Could you check a few things on this model? Use its own coordinates, in mm. Face numbers are marked on the shaded views. Coordinates: 2 decimals unless noted, no trailing zeros. Loops run counter-clockwise (first coordinate to the right, second up) from the corner with the lowest first, then second, coordinate; pieces in that order, holes last.
1) Thinking about a two-plate mould opening in Y: for the marked faces 1, 2, 3 and 4, which applies, released by +Y, released by -Y, zero draft, split by the parting line, or undercut?
2) Imagine slicing it at C-C on x = 53. Please give me the cut outline in (y, z).
3) Imagine slicing it at B-B on z = 4.25. Give the number of separate pieces and of enclosed holes in the cut face, plus the area to 3 significant figures.
4) Will these pins go through, and if not, where does the flat tip stop? P1, Ø3, axis at x = -17.5, y = 19.5, coming from the +Z side; P2, Ø17, axis at x = 53, y = 0, coming from the +Z side.
5) Imagine slicing it at D-D on y = 9. Please give me the cut outline in (x, z), plus the area to 3 significant figures.
6) Imagine slicing it at A-A on y = 0. Please give me the cut outline in (x, z).
7) If I drill on line 1 along X through (y, z) = (-9.5, 6); line 2 along X through (y, z) = (6, 11); line 3 along Y through (x, z) = (1, 7.25), over which ranges is the centre line in solid material (lowest first)?
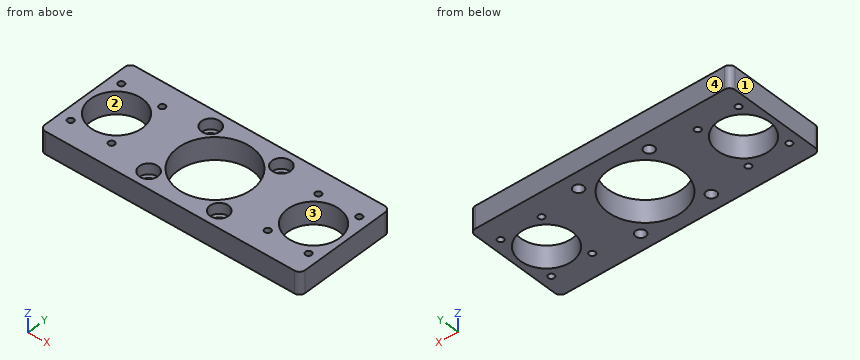
```python
from build123d import *

# Parameters (mm, degrees)
SKETCH_1_W                = 140
SKETCH_1_H                = 55
EXTRUDE_1_DEPTH           = 12
SKETCH_2_R                = 20
SKETCH_2_R_2              = 14
CUT_EXTRUDE_1_DEPTH       = 77.159372371
FILLET_1_R                = 3
HOLE_WIZARD_M4_1_D        = 3.3
HOLE_WIZARD_1_D           = 5.5
HOLE_WIZARD_1_CBORE_D     = 10
HOLE_WIZARD_1_CBORE_DEPTH = 5.7


with BuildPart() as part:
    # 草图1 → 凸台-拉伸1 (new body)
    with BuildSketch(Plane.XY):
        Rectangle(SKETCH_1_W, SKETCH_1_H)
    extrude(amount=EXTRUDE_1_DEPTH)

    # 草图2 → 切除-拉伸1 (cut, through all)
    with BuildSketch(Plane.XY.offset(12)):
        Circle(SKETCH_2_R)
        with Locations((-53, 0)):
            Circle(SKETCH_2_R_2)
        with Locations((53, 0)):
            Circle(SKETCH_2_R_2)
    extrude(amount=-CUT_EXTRUDE_1_DEPTH, mode=Mode.SUBTRACT)

    # 圆角1
    fillet_1_edges = [part.edges().sort_by_distance(p)[0] for p in [
        (70, -27.5, 6),
        (-70, -27.5, 6),
        (-70, 27.5, 6),
        (70, 27.5, 6),
    ]]
    fillet(fillet_1_edges, radius=FILLET_1_R)

    # M4 螺纹孔1 (through all)
    with Locations(Plane.XY.offset(12)):
        with Locations((-64, 15.5), (-42, 15.5), (-42, -15.5), (-64, -15.5), (42, -15.5), (64, -15.5), (64, 15.5), (42, 15.5)):
            Hole(HOLE_WIZARD_M4_1_D / 2)

    # 打孔尺寸(%根据)内六角圆柱头螺钉的类型1 (through all)
    with Locations(Plane.XY.offset(12)):
        with Locations((-19, 19), (19, 19), (19, -19), (-19, -19)):
            CounterBoreHole(HOLE_WIZARD_1_D / 2, HOLE_WIZARD_1_CBORE_D / 2, HOLE_WIZARD_1_CBORE_DEPTH)


solid = part.part
```
Filled in:
1. face 1: zero draft
1. face 2: undercut
1. face 3: undercut
1. face 4: released by +Y
2. outline: (-27.5, 0) - (-14, 0) - (-14, 12) - (-27.5, 12) - close; (14, 0) - (27.5, 0) - (27.5, 12) - (14, 12) - close
3. separate pieces: 1
3. enclosed holes: 15
3. area: 5,040 mm2
4. P1: stops at z = 6.3
4. P2: passes through
5. outline: (-70, 0) - (-63.72, 0) - (-63.72, 12) - (-70, 12) - close; (-42.28, 0) - (-17.86, 0) - (-17.86, 12) - (-42.28, 12) - close; (17.86, 0) - (42.28, 0) - (42.28, 12) - (17.86, 12) - close; (63.72, 0) - (70, 0) - (70, 12) - (63.72, 12) - close
5. area: 737 mm2
6. outline: (-70, 0) - (-67, 0) - (-67, 12) - (-70, 12) - close; (-39, 0) - (-20, 0) - (-20, 12) - (-39, 12) - close; (20, 0) - (39, 0) - (39, 12) - (20, 12) - close; (67, 0) - (70, 0) - (70, 12) - (67, 12) - close
7. line 1: x = -70 to -63.28, -42.72 to -17.6, 17.6 to 42.72, 63.28 to 70
7. line 2: x = -70 to -65.65, -40.35 to -19.08, 19.08 to 40.35, 65.65 to 70
7. line 3: y = -27.5 to -19.97, 19.97 to 27.5
